Autodesk Inventor part; units mm, degrees
ref_plane "YZ Plane" through (0, 0, 0) normal (1, 0, 0) x (0, 1, 0)
ref_plane "XZ Plane" through (0, 0, 0) normal (0, 1, 0) x (-1, 0, 0)
ref_plane "XY Plane" through (0, 0, 0) normal (0, 0, 1) x (1, 0, 0)
sketch "Sketch1" plane through (0, 0, 0) normal (0, 0, 1) x (1, 0, 0)
  line L0 (20.5, -20.5) -> (-20.5, -20.5)
  line L1 (-20.5, -20.5) -> (-20.5, 20.5)
  line L2 (-20.5, 20.5) -> (20.5, 20.5)
  line L3 (20.5, 20.5) -> (20.5, -20.5)
  line L4 (20.5, -20.5) -> (-20.5, 20.5) construction
  line L5 (-20.5, -20.5) -> (20.5, 20.5) construction
  line L6 (22.5, -22.5) -> (-22.5, -22.5)
  line L7 (-22.5, -22.5) -> (-22.5, 22.5)
  line L8 (-22.5, 22.5) -> (22.5, 22.5)
  line L9 (22.5, 22.5) -> (22.5, -22.5)
  line L10 (22.5, -22.5) -> (-22.5, 22.5) construction
  line L11 (-22.5, -22.5) -> (22.5, 22.5) construction
  point P0 (0, 0)
  dimension "d0" = 41
  dimension "d1" = 41
  dimension "d2" = 45
  dimension "d3" = 45
extrude "Extrusion1" add sketch "Sketch1" along normal blind 90
extrude "Extrusion2" add sketch "Sketch1" along normal blind 2.5 contours L0 L1 L2 L3
sketch "Sketch2" plane through (-22.5, 22.5, 0) normal (0, 1, 0) x (1, 0, 0)
  line L0 (0, 0) -> (45, 0)
  line L1 (45, 0) -> (45, -45)
  line L2 (45, -45) -> (0, -45)
  line L3 (0, -45) -> (0, 0)
  line L4 (0, -45) -> (45, 0) construction
  line L5 (45, -45) -> (0, 0) construction
  line L6 (43, -2) -> (2, -2)
  line L7 (2, -2) -> (2, -43)
  line L8 (2, -43) -> (43, -43)
  line L9 (43, -43) -> (43, -2)
  line L10 (43, -2) -> (2, -43) construction
  line L11 (2, -2) -> (43, -43) construction
  line L12 (22.5, -22.5) -> (22.5, -90) construction
  line L13 (43, -90) -> (2, -90) construction
  line L14 (22.5, -90) -> (27.5, -90) construction
  line L15 (27.5, -90) -> (17.5, -90)
  line L16 (17.5, -90) -> (17.5, -45)
  line L17 (17.5, -45) -> (27.5, -45)
  line L18 (27.5, -45) -> (27.5, -90)
  point P0 (22.5, 0)
  dimension "d8" = 45
  dimension "d9" = 45
  dimension "d10" = 41
  dimension "d11" = 41
  dimension "d16" = 5
  dimension "d17" = 10
extrude "Extrusion3" add sketch "Sketch2" along normal blind 45 contours L0 L1 L2 L3
extrude "Extrusion4" cut sketch "Sketch2" against normal blind 40 contours L9 L8 L7 L6
extrude "Extrusion5" add sketch "Sketch2" along normal blind 45 contours L2 L18 L15 L16
chamfer "Chamfer1" distance 45 angle 45 1 edges at (0, 67.5, 90)
sketch "Sketch3" plane through (-22.5, -22.5, 0) normal (0, -1, 0) x (1, 0, 0)
  line L0 (0, 0) -> (0, 90)
  line L1 (45, 45) -> (45, 90) construction
  line L2 (45, 90) -> (0, 90) construction
  line L3 (0, 90) -> (0, 45) construction
  line L4 (0, 45) -> (45, 45) construction
  line L5 (45, 45) -> (45, 90) construction
  line L6 (0, 45) -> (45, 45) construction
  line L7 (45, 45) -> (45, 0) construction
  line L8 (45, 0) -> (0, 0) construction
  line L9 (0, 0) -> (0, 45) construction
  line L10 (0, 45) -> (0, 90) construction
  line L11 (45, 90) -> (0, 45) construction
  line L12 (0, 45) -> (45, 0) construction
  line L13 (45, 0) -> (0, 0) construction
  line L14 (0, 0) -> (45, 45) construction
  line L15 (0, 90) -> (45, 45) construction
  point P0 (22.5, 0)
  point P1 (22.5, 67.5)
  point P2 (22.5, 22.5)
hole "Hole1" at (0, -22.5, 67.5) at (0, -22.5, 22.5) direction (0, 1, 0) diameter 5 depth 8 tip angle 118
sketch "Sketch5" plane through (0, 0, 0) normal (0, 0, -1) x (-1, 0, 0)
  line L0 (22.5, -22.5) -> (22.5, 67.5)
  line L1 (-22.5, -22.5) -> (22.5, -22.5) construction
  line L2 (22.5, -22.5) -> (22.5, 22.5) construction
  line L3 (22.5, 22.5) -> (-22.5, 22.5) construction
  line L4 (-22.5, 22.5) -> (-22.5, -22.5) construction
  line L5 (22.5, 22.5) -> (-22.5, 22.5) construction
  line L6 (-22.5, 22.5) -> (-22.5, 67.5) construction
  line L7 (-22.5, 67.5) -> (22.5, 67.5) construction
  line L8 (22.5, 67.5) -> (22.5, 22.5) construction
  line L9 (-22.5, 22.5) -> (22.5, 67.5) construction
  line L10 (22.5, 22.5) -> (-22.5, 67.5) construction
  point P0 (0, 0)
  point P1 (0, 45)
hole "Hole2" at (0, 45, 0) direction (0, 0, 1) diameter 5 depth 8 tip angle 118
fillet "Fillet1" radius 2.5 15 edges at (-22.5, 45, 45) (-22.5, 22.5, 67.5) (-22.5, -22.5, 45) (-22.5, 22.5, 0) (22.5, 22.5, 67.5) (22.5, 45, 45) (22.5, -22.5, 45) (22.5, 22.5, 0) (0, -22.5, 0) (-5, 22.5, 67.5) (-5, 45, 45) (-13.75, 22.5, 45) (5, 22.5, 67.5) (13.75, 22.5, 45) (5, 45, 45)
properties part number "L_connector"
Geometry: final body of the model. Coordinates: model frame, mm. A direction names the side the tool comes from. Round coordinates to 2 decimals unless told otherwise and drop trailing zeros. Loops run counter-clockwise (first coordinate to the right, second up) from the corner with the lowest first, then second, coordinate; pieces in that order, holes last. Notation, with made-up numbers: M 49.25,-16.5 L 78.25,-16.5 A17 cw 78.25,-9.5 Z; hole C -22,19.25 d6. An arc over 180 degrees is marked long. One line per question, with ' | ' between items.
(1) Cut plane C-C on y = 52. Return the cut outline in (x, z).
Check result:
outline: M -22.5,2.5 A2.5 ccw -20,0 L 20,0 A2.5 ccw 22.5,2.5 L 22.5,42.5 A2.5 ccw 20,45 L 7.5,45 A2.5 cw 5,47.5 L 5,60.5 L -5,60.5 L -5,47.5 A2.5 cw -7.5,45 L -20,45 A2.5 ccw -22.5,42.5 Z; hole M -20.5,2 L 20.5,2 L 20.5,43 L -20.5,43 Z
(2) Contact query for flat-ended pins moving along their axis: P1, Ø4, axis at x = -12.5, y = 43, coming from the +Z side; P2, Ø3, axis at x = 0, z = 67.5, coming from the -Y side; P3, Ø1.5, axis at x = 3, y = -19, coming from the +Z side. Output: stop coordinate, or through.
Check result:
P1: stops at z = 45 | P2: stops at y = 20.5 | P3: stops at z = 2.5
(3) Material intervals for line 1 along X through (y, z) = (4, 68); line 2 along Z through (x, y) = (-17, 57), sorted ascending. Write a range as from..to.
Check result:
line 1: x = -22.5..-20.5, 20.5..22.5 | line 2: z = 0..2, 43..45
(4) Cut plane D-D on z = 84. Return the cut outline in (x, y).
Check result:
outline: M -22.5,-20 A2.5 ccw -20,-22.5 L 20,-22.5 A2.5 ccw 22.5,-20 L 22.5,20 A2.5 ccw 20,22.5 L 7.5,22.5 A2.5 cw 5,25 L 5,28.5 L -5,28.5 L -5,25 A2.5 cw -7.5,22.5 L -20,22.5 A2.5 ccw -22.5,20 Z; hole M -20.5,-20.5 L 20.5,-20.5 L 20.5,20.5 L -20.5,20.5 Z
(5) Cut plane A-A on x = 12. Return the cut outline in (y, z).
Check result:
outline: M -22.5,2.5 A2.5 ccw -20,0 L 67.5,0 L 67.5,2 L -17.5,2 L -17.5,2.5 L -20.5,2.5 L -20.5,90 L -22.5,90 Z; M 20.5,43 L 67.5,43 L 67.5,45 L 25,45 A2.5 cw 22.5,47.5 L 22.5,90 L 20.5,90 Z
(6) Pull-direction query (Y, two-part tool) for faces 1 (the cylindrical face through (14, 23, 46)), 2 (the cylindrical face through (0.96, 47.31, 1.01)), 3 (the cylindrical face through (22, 23, 1)); classes: +Y half, -Y half, draft (parallel to the pull), parting line (faces both ways), or undercut.
Check result:
face 1: +Y half | face 2: undercut | face 3: draft
(7) Cut plane B-B on z = 22.5. Return the cut outline in (x, y).
Check result:
outline: M -22.5,-20 A2.5 ccw -20,-22.5 L -2.5,-22.5 L -2.5,-20.5 L -20.5,-20.5 L -20.5,67.5 L -22.5,67.5 Z; M 2.5,-22.5 L 20,-22.5 A2.5 ccw 22.5,-20 L 22.5,67.5 L 20.5,67.5 L 20.5,-20.5 L 2.5,-20.5 Z
(8) Access query for faces 4 (the flat face through (20.5, 13, 37)), 5 (the flat face through (0, 24, 2)), 6 (the flat face through (0, -20.5, 46)), 7 (the flat face through (-14, 46, 45)). Directions: +Z, -Z, +X, -X, +Y, -Y. A direction counts if a zero-diameter tool reaches every point of the face in a straight line with its end or side. Return the directions, or none.
Check result:
face 4: none | face 5: +Y | face 6: +Z | face 7: +Z, -X, +Y
